Geometry check sheet. Reference: the model listing, model coordinates, mm. A direction names the side the tool comes from. Give positions to 0.01 mm unless a question says otherwise; leave off trailing zeros. Write item = value, one per line.
```python
from build123d import *

# Parameters (mm, degrees)
SKETCH1_R           = 63
BOSS_EXTRUDE1_DEPTH = 6
CHAMFER2_SIZE       = 1
SKETCH4_W           = 52.5
SKETCH4_H           = 30.8
SKETCH4_W_2         = 42.5
SKETCH4_H_2         = 20.8
BOSS_EXTRUDE2_DEPTH = 10
SKETCH5_W           = 5
SKETCH5_H           = 8
CUT_EXTRUDE1_DEPTH  = 7.6
SKETCH6_R           = 1.15
CUT_EXTRUDE2_DEPTH  = 90.654893899
SKETCH7_R           = 2.1
CUT_EXTRUDE3_DEPTH  = 4.41
CHAMFER3_SIZE       = 1
CHAMFER4_SIZE       = 0.5


with BuildPart() as part:
    # Sketch1 → Boss-Extrude1 (new body)
    with BuildSketch(Plane(origin=(0, 0, 0), x_dir=(1, 0, 0), z_dir=(0, 1, 0))):
        with Locations(Location((0, 0, 0), (0, 0, 270))):
            Circle(SKETCH1_R)
    extrude(amount=BOSS_EXTRUDE1_DEPTH)

    # Chamfer2
    chamfer2_edges = [part.edges().sort_by_distance(p)[0] for p in [
        (0, 0, -63),
        (0, 6, -63),
    ]]
    chamfer(chamfer2_edges, length=CHAMFER2_SIZE)

    # Sketch4 → Boss-Extrude2 (add)
    with BuildSketch(Plane(origin=(0, 6, 0), x_dir=(1, 0, 0), z_dir=(0, 1, 0))):
        with Locations((-10.25, 0)):
            Rectangle(SKETCH4_W, SKETCH4_H)
        with Locations((-10.25, 0)):
            Rectangle(SKETCH4_W_2, SKETCH4_H_2, mode=Mode.SUBTRACT)
    extrude(amount=BOSS_EXTRUDE2_DEPTH)

    # Sketch5 → Cut-Extrude1 (cut)
    with BuildSketch(Plane(origin=(0, 16, 0), x_dir=(1, 0, 0), z_dir=(0, 1, 0))):
        with Locations((13.5, 0)):
            Rectangle(SKETCH5_W, SKETCH5_H)
    extrude(amount=-CUT_EXTRUDE1_DEPTH, mode=Mode.SUBTRACT)

    # Sketch6 → Cut-Extrude2 (cut, through all)
    with BuildSketch(Plane(origin=(0, 6, 0), x_dir=(1, 0, 0), z_dir=(0, 1, 0))):
        with Locations(Location((-28.35, 7.7, 0), (0, 0, 270))):
            Circle(SKETCH6_R)
        with Locations(Location((7.85, 7.7, 0), (0, 0, 90))):
            Circle(SKETCH6_R)
        with Locations(Location((7.85, -7.7, 0), (0, 0, 270))):
            Circle(SKETCH6_R)
        with Locations(Location((-28.35, -7.7, 0), (0, 0, 90))):
            Circle(SKETCH6_R)
    extrude(amount=-CUT_EXTRUDE2_DEPTH, mode=Mode.SUBTRACT)

    # Sketch7 → Cut-Extrude3 (cut)
    with BuildSketch(Plane.XZ):
        with Locations(Location((-28.35, 7.7, 0), (0, 0, 270))):
            Circle(SKETCH7_R)
        with Locations(Location((7.85, 7.7, 0), (0, 0, 270))):
            Circle(SKETCH7_R)
        with Locations(Location((-28.35, -7.7, 0), (0, 0, 270))):
            Circle(SKETCH7_R)
        with Locations(Location((7.85, -7.7, 0), (0, 0, 270))):
            Circle(SKETCH7_R)
    extrude(amount=-CUT_EXTRUDE3_DEPTH, mode=Mode.SUBTRACT)

    # Chamfer3
    chamfer3_edges = [part.edges().sort_by_distance(p)[0] for p in [
        (16, 16, 9.7),
        (-10.25, 16, -15.4),
        (-36.5, 16, 0),
        (-10.25, 16, 15.4),
        (16, 6, 0),
        (16, 11, 15.4),
        (-10.25, 6, -15.4),
        (16, 11, -15.4),
        (-36.5, 6, 0),
        (-36.5, 11, -15.4),
        (-10.25, 6, 15.4),
        (-36.5, 11, 15.4),
        (11, 16, 7.2),
        (-10.25, 16, -10.4),
        (-31.5, 16, 0),
        (-10.25, 16, 10.4),
        (11, 16, -7.2),
        (16, 16, -9.7),
        (16, 8.4, 0),
        (16, 12.2, -4),
        (16, 12.2, 4),
        (11, 8.4, 0),
        (11, 12.2, 4),
        (11, 12.2, -4),
        (13.5, 16, -4),
        (13.5, 16, 4),
    ]]
    chamfer(chamfer3_edges, length=CHAMFER3_SIZE)

    # Chamfer4
    chamfer4_edges = [part.edges().sort_by_distance(p)[0] for p in [
        (7.85, 0, 9.8),
        (-28.35, 0, -5.6),
        (7.85, 0, -5.6),
        (-28.35, 0, 9.8),
    ]]
    chamfer(chamfer4_edges, length=CHAMFER4_SIZE)


solid = part.part
```
Item 1: Gauge pin test, flat ends, axial feed: pin 1 (1.3 mm diameter, centred on x = 8, z = 7, fed in from -Y); pin 2 (2.5 mm diameter, centred on y = 9, z = 2.5, fed in from -X); pin 3 (7 mm diameter, centred on y = 10, z = 1.5, fed in from +X). Record the tip position at first contact, or that the pin passes through.
Answer:
pin_1 = 4.41
pin_2 = -36.5
pin_3 = 16.5
Item 2: Draft check along X on faces 1 (the flat face through (-29.3, 4.41, 6.8)), 2 (the flat face through (-10, 16, 12)), 3 (the flat face through (16, 11, -6)). Enter one of: +X half, -X half, draft (parallel to the pull), parting line (faces both ways), or undercut.
Answer:
face_1 = undercut
face_2 = draft
face_3 = +X half
Item 3: Thickness scan on L1, parallel to Z at x = 1.5, y = 10.5; L2, parallel to X at y = 5.2, z = 7.7; L3, parallel to Y at x = -3, z = -43.5. Record the ranges inside material, lowest first. Write a range as [from, to].
Answer:
L1 = [-15.4, -10.4], [10.4, 15.4]
L2 = [-62.33, -29.5], [-27.2, 6.7], [9, 62.33]
L3 = [0, 6]
Item 4: Tool access check on faces 4 (the flat face through (-11, 10, 10.4)), 5 (the flat face through (13, 8.4, 0)), 6 (the cylindrical face through (-26.58, 2.43, -8.83)). Record the directions out of +Z, -Z, +X, -X, +Y, -Y that give a thin tool (end or side, any length) a straight path to the whole face; none if there is none.
Answer:
face_4 = +Y
face_5 = +X, +Y
face_6 = -Y
